Could you check a few things on this model? Use its own coordinates, in mm. A direction names the side the tool comes from. Give positions to 0.01 mm unless a question says otherwise; leave off trailing zeros. Loops run counter-clockwise (first coordinate to the right, second up) from the corner with the lowest first, then second, coordinate; pieces in that order, holes last. Notation, with made-up numbers: M -24.5,54.25 L 31.5,54.25 A14 ccw 31.5,67.25 Z; hole C 74,20.5 d8. An arc over 180 degrees is marked long. Answer in a Markdown table with one row per item. Add a question column.
1. I need wall thicknesses on line 1 along Y through (x, z) = (0.85, 2.55); line 2 along X through (y, z) = (-2.5, -1.3); line 3 along Z through (x, y) = (0.45, -4.5). Which ranges of each line are inside material? Lowest first, please. Write a range as from..to.
2. If we section it at B-B on x = 0: List the corners of the cut face in (y, z) for me, then the cut area to 3 significant figures.
3. I'm going to push flat-ended pins straight in: pin 1 Ø2 at (y, z) = (-3.5, 0) entering from +X; pin 2 Ø3 at (x, y) = (-0.5, -5.5) entering from -Z. Where does each tip first touch, or does it pass through?
4. If we section it at C-C on y = -8: List the corners of the cut face in (x, z) for me.
5. If we section it at A-A on z = 0: List the corners of the cut face in (x, y) for me, then the cut area to 3 significant figures.
6. Which directions (+Z, -Z, +X, -X, +Y, -Y) give clear straight access to the entire face, cutting with the end or side of a thin tool? Please do faces 1 (the cylindrical face through (-1.825, -4.437, -1.4)), 2 (the cylindrical face through (-3, 1, 0)).
```python
from build123d import *

# Parameters (mm, degrees)
SKETCH1_R           = 3
BOSS_EXTRUDE1_DEPTH = 3
FILLET1_R           = 0.5
SKETCH2_R           = 2.3
BOSS_EXTRUDE2_DEPTH = 9


with BuildPart() as part:
    # Sketch1 → Boss-Extrude1 (new body)
    with BuildSketch(Plane(origin=(0, 0, 0), x_dir=(1, 0, 0), z_dir=(0, 1, 0))):
        Circle(SKETCH1_R)
    extrude(amount=BOSS_EXTRUDE1_DEPTH)

    # Fillet1
    fillet1_edges = [part.edges().sort_by_distance(p)[0] for p in [
        (-3, 3, 0),
    ]]
    fillet(fillet1_edges, radius=FILLET1_R)

    # Sketch2 → Boss-Extrude2 (add)
    with BuildSketch(Plane.XZ):
        Circle(SKETCH2_R)
    extrude(amount=BOSS_EXTRUDE2_DEPTH)


solid = part.part
```
Results:
| question | item | result |
|---|---|---|
| 1 | line 1 | 0..2.96 |
| 1 | line 2 | -1.9..1.9 |
| 1 | line 3 | -2.26..2.26 |
| 2 | outline | M -9,-2.3 L 0,-2.3 L 0,-3 L 2.5,-3 A0.5 ccw 3,-2.5 L 3,2.5 A0.5 ccw 2.5,3 L 0,3 L 0,2.3 L -9,2.3 Z |
| 2 | area | 59.3 mm2 |
| 3 | pin 1 | x = 2.3 |
| 3 | pin 2 | z = -2.3 |
| 4 | outline | C 0,0 d4.6 |
| 5 | outline | M -3,0 L -2.3,0 L -2.3,-9 L 2.3,-9 L 2.3,0 L 3,0 L 3,2.5 A0.5 ccw 2.5,3 L -2.5,3 A0.5 ccw -3,2.5 Z |
| 5 | area | 59.3 mm2 |
| 6 | face 1 | -Y |
| 6 | face 2 | +Y, -Y |
